Can you work these out from the drawing? Everything is in mm from the part's minimum corner. Give positions to 0.01 mm unless a question says otherwise; leave off trailing zeros. Order: outer loops, then holes, each group sorted by start corner. A loop starts at its lowest first (then second) coordinate and runs counter-clockwise, first axis right, second up. Notation, with made-up numbers: M 69.25,52 L 121.25,52 A26 cw 121.25,90 Z; hole C 76,89 d8. An arc over 180 degrees is marked long. Answer as a JSON object with one key per item and string values.
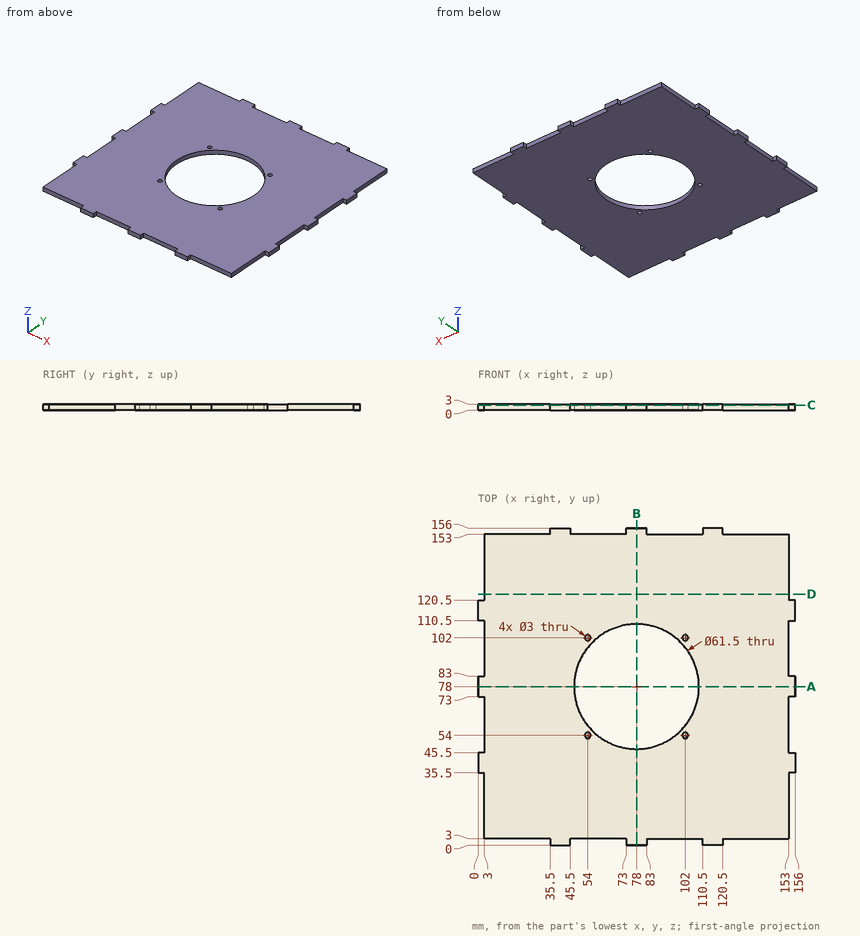
1) I need wall thicknesses on L1, parallel to Y at x = 54, z = 0.8; L2, parallel to X at y = 101, z = 2.85. Which ranges of each line are inside material? Lowest first, please.
Results found:
{"L1": "y = 3 to 52.5, 55.5 to 58.78, 97.22 to 100.5, 103.5 to 153", "L2": "x = 3 to 52.88, 55.12 to 57.59, 98.41 to 100.88, 103.12 to 153"}
2) I want a section at C-C on z = 2.45. Count the separate pieces of the cut face and the enclosed holes in it, and give its area (3 significant figures).
Results found:
{"separate pieces": "1", "enclosed holes": "5", "area": "19,900 mm²"}
3) I want a section at A-A on y = 78. Write out the boundary of the cut face in (x, z), and give its area (4 significant figures).
Results found:
{"outline": "M 0,0 L 47.25,0 L 47.25,3 L 0,3 Z; M 108.75,0 L 156,0 L 156,3 L 108.75,3 Z", "area": "283.5 mm²"}
4) I'm going to push flat-ended pins straight in: pin 1 Ø1.5 at (y, z) = (56.5, 2) entering from +X; pin 2 Ø5 at (x, y) = (54, 102) entering from +Z; pin 3 Ø1.5 at (x, z) = (96, 0.5) entering from -Y; pin 4 Ø1.5 at (y, z) = (1, 2) entering from -X. Where does each tip first touch, or does it pass through?
Results found:
{"pin 1": "stops at x = 153", "pin 2": "stops at z = 3", "pin 3": "stops at y = 3", "pin 4": "stops at x = 35.5"}
5) I want a section at D-D on y = 123.5. Write out the boundary of the cut face in (x, z).
Results found:
{"outline": "M 3,0 L 153,0 L 153,3 L 3,3 Z"}
